Autodesk Inventor part; units mm, degrees
ref_plane "YZ Plane" through (0, 0, 0) normal (1, 0, 0) x (0, 1, 0)
ref_plane "XZ Plane" through (0, 0, 0) normal (0, 1, 0) x (-1, 0, 0)
ref_plane "XY Plane" through (0, 0, 0) normal (0, 0, 1) x (1, 0, 0)
sketch "Sketch3" plane through (0, 0, 0) normal (0, 0, 1) x (1, 0, 0)
  line L0 (51.7998, 73.9071) -> (77.1998, 73.9071)
  line L1 (77.1998, 73.9071) -> (77.1998, 48.5071)
  line L2 (77.1998, 48.5071) -> (51.7998, 48.5071)
  line L3 (51.7998, 48.5071) -> (51.7998, 73.9071)
  point P0 (0, 0)
  dimension "d2" = 25.4
  dimension "d3" = 25.4
extrude "Extrusion2" add sketch "Sketch3" along normal blind 17.78
sketch "Sketch4" plane through (0, 0, 17.78) normal (0, 0, 1) x (1, 0, 0)
  circle A0 centre (64.4141, 63.8936) radius 4.6626
  point P0 (0, 0)
extrude "Extrusion3" add sketch "Sketch4" along normal blind 50.8
properties part number "galvo"
Geometry check sheet. Reference: the model listing, model coordinates, mm. A direction names the side the tool comes from. Round coordinates to 2 decimals unless told otherwise and drop trailing zeros. Write each loop counter-clockwise with the first axis right and the second up, starting at its lowest first coordinate (ties: lowest second). Pieces come first, ordered by that corner, then holes. Notation, with made-up numbers: (86.25, 67.5) -> (122.25, 67.5) arc R23 cw to (122.25, 80.5) -> close; hole circle Ø1 at (89.25, -21). An arc over 180 degrees is marked (long way). One line per item, written item: value. Start each with the question number.
(1) Cross-section at D-D, the plane z = 60.5. Record the cut outline in (x, y).
(2) Cross-section at C-C, the plane x = 57.5. Record the cut outline in (y, z).
(3) Access from +Z, -Z, +X, -X, +Y, -Y to the whole of each face (thin tool, end or side, straight path). Record for faces 1 (the cylindrical face through (66.57, 68.03, 42.82)), 2 (the flat face through (64, 73.907, 9)).
(4) Scan lines: line 1 (Z direction, x = 53, y = 53.5); line 2 (X direction, y = 63.5, z = 39); line 3 (X direction, y = 64.5, z = 23). Record each from-to range of solid material in increasing order. Write a range as [from, to].
(5) Cross-section at B-B, the plane y = 57. Record the cut outline in (x, z), and give its area (3 significant figures).
(6) Cross-section at A-A, the plane x = 67.75. Record the cut outline in (y, z), and give its area (3 significant figures).
(7) Go/stop test with flat-tipped pins: pin 1 Ø3 at (x, y) = (58.5, 58) entering from +Z; pin 2 Ø5 at (x, y) = (57.5, 51.5) entering from -Z; pin 3 Ø1.5 at (x, z) = (68.5, 53) entering from +Y. Record where each tip stops, or that it passes through.
Answer:
1. outline: circle Ø9.33 at (64.41, 63.89)
2. outline: (48.51, 0) -> (73.91, 0) -> (73.91, 17.78) -> (48.51, 17.78) -> close
3. face 1: +Z
3. face 2: +Z, -Z, +X, -X, +Y
4. line 1: [0, 17.78]
4. line 2: [59.77, 69.06]
4. line 3: [59.79, 69.04]
5. outline: (51.8, 0) -> (77.2, 0) -> (77.2, 17.78) -> (51.8, 17.78) -> close
5. area: 452 mm²
6. outline: (48.51, 0) -> (73.91, 0) -> (73.91, 17.78) -> (67.15, 17.78) -> (67.15, 68.58) -> (60.64, 68.58) -> (60.64, 17.78) -> (48.51, 17.78) -> close
6. area: 783 mm²
7. pin 1: z = 17.78
7. pin 2: z = 0
7. pin 3: y = 67.15
